Source: CAD feature listing. Evaluate the final solid. Frame: model axes, mm. A direction names the side the tool comes from. Coordinates: 2 decimals unless noted, no trailing zeros. Order: outer loops, then holes, each group sorted by start corner. A loop starts at its lowest first (then second) coordinate and runs counter-clockwise, first axis right, second up.
Autodesk Inventor part; units mm, degrees
ref_plane "Work Plane1" through (0, 0, 10.7) normal (0, 0, 1) x (1, 0, 0)
ref_plane "YZ Plane" through (0, 0, 0) normal (1, 0, 0) x (0, 1, 0)
ref_plane "XZ Plane" through (0, 0, 0) normal (0, 1, 0) x (-1, 0, 0)
sketch "Sketch1" plane through (0, 0, 0) normal (0, 0, 1) x (1, 0, 0)
  line L0 (-10.4, -2.75) -> (10.4, -2.75)
  line L1 (10.4, -2.75) -> (10.4, 2.75)
  line L2 (10.4, 2.75) -> (-10.4, 2.75)
  line L3 (-10.4, 2.75) -> (-10.4, -2.75)
  point P0 (0, 0)
  dimension "d268" = 5.5
  dimension "d269" = 2.75
  dimension "d270" = 20.8
  dimension "d271" = 10.4
extrude "Extrusion1" add sketch "Sketch1" along normal blind 10.2
sketch "Sketch2" plane through (-6.98, -2.75, 0) normal (0, -1, 0) x (1, 0, 0)
  line L0 (0, 0) -> (13.96, 0)
  line L1 (5.18, 3.6) -> (8.78, 3.6)
  line L2 (8.78, 3.6) -> (8.78, 0.5)
  line L3 (8.28, 0) -> (5.68, 0)
  line L4 (5.18, 0.5) -> (5.18, 3.6)
  line L5 (5.18, 0.5) -> (5.68, 0)
  line L6 (8.78, 0.5) -> (8.28, 0)
  point P0 (6.98, 0)
  dimension "d15" = 3.6
  dimension "d17" = 0.5
  dimension "d19" = 135
  dimension "d20" = 135
  dimension "d21" = 0.5
  dimension "d22" = 3.6
extrude "Extrusion2" [suppressed]
sketch "Sketch3" plane through (0, 0, 0) normal (0, 1, 0) x (-1, 0, 0)
  line L0 (-6.98, 3.6) -> (-7.23, 3.6)
  line L1 (-7.98, 2.1) -> (-7.98, 1.22)
  line L2 (-7.98, 1.22) -> (-6.98, 1.22)
  line L3 (-6.98, 1.22) -> (-6.98, 3.6)
  line L4 (6.98, 10.2) -> (-6.98, 10.2)
  line L5 (0, 10.2) -> (0, 0)
  line L6 (-6.98, 0) -> (6.98, 0)
  line L7 (-7.23, 3.6) -> (-7.98, 2.1)
  line L8 (6.98, 3.6) -> (7.23, 3.6)
  line L9 (7.98, 2.1) -> (7.98, 1.22)
  line L10 (7.98, 1.22) -> (6.98, 1.22)
  line L11 (6.98, 1.22) -> (6.98, 3.6)
  line L12 (7.23, 3.6) -> (7.98, 2.1)
  dimension "d25" = 13.96
  dimension "d26" = 1.22
  dimension "d28" = 1
  dimension "d29" = 1.5
  dimension "d30" = 0.88
  dimension "d31" = 0.25
extrude "Extrusion3" [suppressed]
sketch "Sketch4" plane through (0, -0.5, 0) normal (0, -1, 0) x (1, 0, 0)
  line L0 (6.98, 3.6) -> (7.23, 3.6)
  line L1 (6.98, 6.263) -> (7.23, 6.263)
  line L2 (7.98, 5.513) -> (7.98, 5.263)
  line L3 (7.98, 5.263) -> (6.98, 5.263)
  line L4 (6.98, 5.263) -> (6.98, 6.263)
  line L5 (-6.98, 10.2) -> (6.98, 10.2)
  line L6 (6.98, 0) -> (-6.98, 0)
  line L7 (0, 10.2) -> (0, 0)
  line L8 (7.23, 6.263) -> (7.98, 5.513)
  line L9 (-6.98, 6.263) -> (-7.23, 6.263)
  line L10 (-7.98, 5.513) -> (-7.98, 5.263)
  line L11 (-7.98, 5.263) -> (-6.98, 5.263)
  line L12 (-6.98, 5.263) -> (-6.98, 6.263)
  line L13 (-7.23, 6.263) -> (-7.98, 5.513)
  dimension "d34" = 1.663
  dimension "d35" = 13.96
  dimension "d36" = 1
  dimension "d38" = 0.25
  dimension "d39" = 1
  dimension "d40" = 0.25
extrude "Extrusion4" [suppressed]
sketch "Sketch5" plane through (0, 0.5, 0) normal (0, 1, 0) x (1, 0, 0)
  line L0 (7.23, -3.6) -> (6.98, -3.6)
  line L1 (7.23, -6.263) -> (6.98, -6.263)
  line L2 (6.98, -6.263) -> (6.98, -5.263)
  line L3 (6.98, -5.263) -> (7.98, -5.263)
  line L4 (7.98, -5.263) -> (7.98, -5.513)
  line L5 (6.98, -10.2) -> (-6.98, -10.2)
  line L6 (1.3, 0) -> (-1.3, 0)
  line L7 (0, 0) -> (0, -10.2)
  line L8 (7.23, -6.263) -> (7.98, -5.513)
  line L9 (-7.23, -6.263) -> (-6.98, -6.263)
  line L10 (-6.98, -6.263) -> (-6.98, -5.263)
  line L11 (-6.98, -5.263) -> (-7.98, -5.263)
  line L12 (-7.98, -5.263) -> (-7.98, -5.513)
  line L13 (-7.23, -6.263) -> (-7.98, -5.513)
  dimension "d43" = 1.663
  dimension "d44" = 13.96
  dimension "d45" = 1
  dimension "d46" = 1
  dimension "d47" = 0.25
  dimension "d48" = 0.25
extrude "Extrusion5" [suppressed]
sketch "Sketch6" plane through (-6.98, -2.75, 10.2) normal (0, -1, 0) x (1, 0, 0)
  line L0 (0, -10.2) -> (5.68, -10.2)
  line L1 (-38.97, -10.2) -> (-36.97, -6.7359)
  line L2 (-36.97, -6.7359) -> (-34.97, -10.2)
  line L3 (-38.97, -10.2) -> (-34.97, -10.2)
  line L4 (0.5, -10.2) -> (2.5, -6.7359)
  line L5 (2.5, -6.7359) -> (4.5, -10.2)
  line L6 (0.5, -10.2) -> (4.5, -10.2)
  dimension "d61" = 0.5
  dimension "d62" = 4
extrude "Extrusion6" [suppressed]
sketch "Sketch7" plane through (0, 0, 0) normal (0, 0, -1) x (-1, 0, 0)
  line L0 (6.98, 2.75) -> (6.98, -1.25)
  line L1 (4.705, 1.645) -> (5.455, 1.645)
  line L2 (5.455, 1.645) -> (5.455, 0.895)
  line L3 (5.455, 0.895) -> (4.705, 0.895)
  line L4 (4.705, 0.895) -> (4.705, 1.645)
  line L5 (4.705, -0.895) -> (5.455, -0.895)
  line L6 (5.455, -0.895) -> (5.455, -1.645)
  line L7 (5.455, -1.645) -> (4.705, -1.645)
  line L8 (4.705, -1.645) -> (4.705, -0.895)
  line L9 (5.08, 0.895) -> (5.08, -0.895) construction
  point P0 (0, 0)
  point P1 (5.08, 0)
  dimension "d65" = 0.75
  dimension "d66" = 2.54
  dimension "d67" = 1.525
extrude "Extrusion7" [suppressed]
chamfer "Chamfer1" [suppressed]
pattern_linear "Rectangular Pattern1" [suppressed]
ref_plane "Work Plane1" through (0, 0, 10.7) normal (0, 0, 1) x (1, 0, 0)
sketch "Sketch8" plane through (0, 0, 10.7) normal (0, 0, 1) x (1, 0, 0)
  line L0 (-6.98, 2.75) -> (6.98, 2.75)
  line L1 (-6.98, -2.75) -> (-6.98, 2.75)
  line L2 (6.98, -2.75) -> (-6.98, -2.75)
  line L3 (6.98, 2.75) -> (6.98, -2.75)
  line L4 (-7.11, 0) -> (-42.9538, 0)
  line L5 (-10.4, -2.75) -> (-10.4, 2.75)
  line L6 (10.4, -2.75) -> (-10.4, -2.75)
  line L7 (10.4, 2.75) -> (10.4, -2.75)
  line L8 (-10.4, 2.75) -> (10.4, 2.75)
  line L9 (10.4, 2.75) -> (-10.4, 2.75)
  line L10 (10.4, -2.75) -> (-10.4, -2.75)
  line L11 (-10.4, -2.75) -> (-10.4, 2.75)
  line L12 (-10.4, 2.75) -> (10.4, 2.75)
  line L13 (10.4, 2.75) -> (10.4, -2.75)
extrude "Extrusion20" add sketch "Sketch8" along normal blind 0.8
sketch "Sketch22" plane through (0, 0, 0) normal (0, 0, -1) x (-1, 0, 0)
  line L0 (-7.99, -3) -> (-8.665, -3)
  line L1 (8.665, 2.75) -> (-8.665, 2.75)
  line L2 (-8.665, -3) -> (8.665, -3)
  line L3 (8.665, -3) -> (8.665, 2.75)
  line L4 (8.665, 2.75) -> (-8.665, 2.75)
  line L5 (-8.665, 2.75) -> (-8.665, -3)
  point P0 (0, 0)
extrude "Extrusion17" [suppressed]
sketch "Sketch25" plane through (0, 0, 0) normal (0, 0, -1) x (-1, 0, 0)
  line L0 (10.4, -2.75) -> (-10.4, -2.75)
  line L1 (10.4, 2.75) -> (10.4, -2.75)
  line L2 (-10.4, 2.75) -> (10.4, 2.75)
  line L3 (-10.4, -2.75) -> (-10.4, 2.75)
  line L4 (10.4, -2.75) -> (-10.4, -2.75)
  line L5 (-10.4, -2.75) -> (-10.4, 2.75)
  line L6 (-10.4, 2.75) -> (10.4, 2.75)
  line L7 (10.4, 2.75) -> (10.4, -2.75)
  point P0 (0, 0)
extrude "Extrusion21" cut sketch "Sketch25" against normal blind 9.1
sketch "Sketch26" plane through (0, 0, 10.2) normal (0, 0, 1) x (1, 0, 0)
  line L0 (10.4, -2.75) -> (-10.4, -2.75)
  line L1 (10.4, 2.75) -> (-10.4, 2.75)
  line L2 (-10.4, -2.75) -> (-9.4, -2.75)
  line L3 (-9.4, -2.75) -> (-9.4, 2.75)
  line L4 (-9.4, 2.75) -> (-10.4, 2.75)
  line L5 (-10.4, 2.75) -> (-10.4, -2.75)
  point P0 (0, 0)
  dimension "d276" = 1
extrude "Extrusion22" add sketch "Sketch26" along normal blind 0.5
mirror "Mirror1" about plane through (0, 0, 0) normal (1, 0, 0) of "Extrusion22"
equation "\"DimA\" = 13.96"
equation "\"DimB\" = 17.33"
equation "\"DimC\" = 5.715"
properties part number "RC CON_10CKT"
Q1. Pull-direction query (Z, two-part tool) for faces 3 (the flat face through (0, 0, 11.5)), 4 (the flat face through (0, 0, 10.7)), 5 (the flat face through (0, 0, 9.1)), 6 (the flat face through (0, -2.75, 10)); classes: pulls with the +Z half, pulls with the -Z half, needs draft (parallel to the pull), parting line crosses it, or undercut.
Solutions:
face 3: pulls with the +Z half
face 4: undercut
face 5: pulls with the -Z half
face 6: needs draft
Q2. Section query A-A on x = 2.5. Output: boundary loops of the cut face in (y, z), plus the area to 4 significant figures.
Solutions:
outline: (-2.75, 9.1) - (2.75, 9.1) - (2.75, 10.2) - (-2.75, 10.2) - close; (-2.75, 10.7) - (2.75, 10.7) - (2.75, 11.5) - (-2.75, 11.5) - close
area: 10.45 mm2
Q3. Material intervals for line 1 along Z through (x, y) = (-0.75, 0); line 2 along X through (y, z) = (-0.65, 10.4), sorted ascending.
Solutions:
line 1: z = 9.1 to 10.2, 10.7 to 11.5
line 2: x = -10.4 to -9.4, 9.4 to 10.4
Q4. Set-up query: faces 1 (the flat face through (0, 2.75, 10)), 2 (the flat face through (0, 0, 10.2)). Return all of +Z, -Z, +X, -X, +Y, -Y with unobstructed straight access to the full face (end or side cutting, diameter ignored); none if empty.
Solutions:
face 1: +Z, -Z, +X, -X, +Y
face 2: +Y, -Y
Q5. Section query B-B on y = -0.25. Output: boundary loops of the cut face in (x, z), plus the area to 3 significant figures.
Solutions:
outline: (-10.4, 9.1) - (10.4, 9.1) - (10.4, 11.5) - (-10.4, 11.5) - close; hole (-9.4, 10.2) - (9.4, 10.2) - (9.4, 10.7) - (-9.4, 10.7) - close
area: 40.5 mm2
